The listing builds one solid part. Answer for the finished solid, in the listing's coordinates (mm). Face numbers are marked on the shaded views. A direction names the side the tool comes from. Give positions to 0.01 mm unless a question says otherwise; leave off trailing zeros. Order: outer loops, then holes, each group sorted by start corner. A loop starts at its lowest first (then second) coordinate and runs counter-clockwise, first axis right, second up. Notation, with made-up numbers: (51.5, 6.25) - (96.5, 6.25) arc R18 ccw to (96.5, 27.25) - close; hole circle Ø5 at (29, -26). An arc over 180 degrees is marked (long way). Answer as CSV lines item,"result". Start each with the question number.
1. Section D-D on x = 0.45 is taken. Give the vertices of the cut face in (y, z), and give its area (3 significant figures).
2. Section C-C on y = -2.5 is taken. Give the vertices of the cut face in (x, z), and give its area (3 significant figures).
3. Which of the six approach directions +Z, -Z, +X, -X, +Y, -Y give full straight-line access (tool end or side, diameter ignored) to the marked faces 1, 2, 3, 4 and 5?
4. Section B-B on x = 1.1 is taken. Give the vertices of the cut face in (y, z), and give its area (3 significant figures).
5. Consider line 1 along Z through (x, y) = (-0.7, -2.5); line 2 along Y through (x, z) = (-0.9, 2.95); line 3 along X through (y, z) = (3.5, 1.4). Determine where each line is inside the solid, lowest interval first. Write a range as [from, to].
6. Flat-ended cylindrical pins translate along their axes: pin 1 (0.8 mm diameter, centred on y = -3, z = 1.5, fed in from -X); pin 2 (1.2 mm diameter, centred on x = 0.5, y = 3, fed in from -Z); pin 3 (0.8 mm diameter, centred on y = 3, z = 1.5, fed in from +X). Find the tip coordinate at first contact, or state that the pin passes through.
7. Section A-A on z = 0.85 is taken. Give the vertices of the cut face in (x, y), and give its area (3 significant figures).
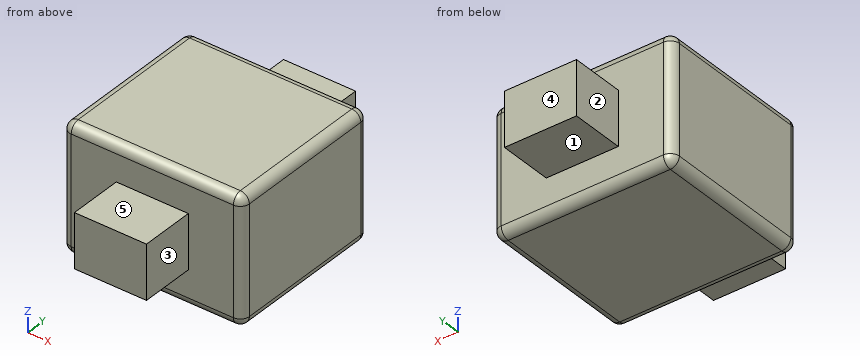
from build123d import *

# Parameters (mm, degrees)
SKETCH1_W           = 5
SKETCH1_H           = 4.5
BOSS_EXTRUDE1_DEPTH = 3.5
BOSS_EXTRUDE2_DEPTH = 1.5
BOSS_EXTRUDE3_DEPTH = 1.5
FILLET1_R           = 0.25


with BuildPart() as part:
    # Sketch1 → Boss-Extrude1 (new body)
    with BuildSketch(Plane.XY):
        Rectangle(SKETCH1_W, SKETCH1_H)
    extrude(amount=BOSS_EXTRUDE1_DEPTH)

    # Sketch2 → Boss-Extrude2 (add)
    with BuildSketch(Plane(origin=(0, 2.25, 0), x_dir=(1, 0, 0), z_dir=(0, 1, 0))):
        Polygon((-1, -2.45), (1, -1.05), (1, -1), (-1, -1), align=None)
        Polygon((1, -2.5), (1, -1.05), (-1, -2.45), (-1, -2.5), align=None)
    extrude(amount=BOSS_EXTRUDE2_DEPTH)

    # Sketch3 → Boss-Extrude3 (add)
    with BuildSketch(Plane(origin=(0, -2.25, 0), x_dir=(-1, 0, 0), z_dir=(0, -1, 0))):
        Polygon((-1, -1), (-1, -2.45), (1, -1.05), (1, -1), align=None)
        Polygon((1, -1.05), (-1, -2.45), (-1, -2.5), (1, -2.5), align=None)
    extrude(amount=BOSS_EXTRUDE3_DEPTH)

    # Fillet1
    fillet1_edges = [part.edges().sort_by_distance(p)[0] for p in [
        (-2.5, 0, 3.5),
        (0, -2.25, 3.5),
        (2.5, 0, 3.5),
        (0, -2.25, 0),
        (-2.5, 0, 0),
        (0, 2.25, 0),
        (2.5, 0, 0),
        (0, 2.25, 3.5),
        (2.5, -2.25, 1.75),
        (-2.5, -2.25, 1.75),
        (-2.5, 2.25, 1.75),
        (2.5, 2.25, 1.75),
    ]]
    fillet(fillet1_edges, radius=FILLET1_R)


solid = part.part
Checks:
1,outline,"(-3.75, 1) - (-2.25, 1) - (-2.25, 0.25) arc R0.25 ccw to (-2, 0) - (2, 0) arc R0.25 ccw to (2.25, 0.25) - (2.25, 1) - (3.75, 1) - (3.75, 2.5) - (2.25, 2.5) - (2.25, 3.25) arc R0.25 ccw to (2, 3.5) - (-2, 3.5) arc R0.25 ccw to (-2.25, 3.25) - (-2.25, 2.5) - (-3.75, 2.5) - close"
1,area,"20.2 mm²"
2,outline,"(-1, 1) - (1, 1) - (1, 2.5) - (-1, 2.5) - close"
2,area,"3.00 mm²"
3,face 1,"-Z, +X, -X, +Y"
3,face 2,"+Z, -Z, -X, +Y"
3,face 3,"+Z, -Z, +X, -Y"
3,face 4,"+Z, -Z, +X, -X, +Y"
3,face 5,"+Z, +X, -X, -Y"
4,outline,"(-2.25, 0.25) arc R0.25 ccw to (-2, 0) - (2, 0) arc R0.25 ccw to (2.25, 0.25) - (2.25, 3.25) arc R0.25 ccw to (2, 3.5) - (-2, 3.5) arc R0.25 ccw to (-2.25, 3.25) - close"
4,area,"15.7 mm²"
5,line 1,"z = [1, 2.5]"
5,line 2,"y = [-2.25, 2.25]"
5,line 3,"x = [-1, 1]"
6,pin 1,"stops at x = -1"
6,pin 2,"stops at z = 1"
6,pin 3,"stops at x = 1"
7,outline,"(-2.5, -2) arc R0.25 ccw to (-2.25, -2.25) - (2.25, -2.25) arc R0.25 ccw to (2.5, -2) - (2.5, 2) arc R0.25 ccw to (2.25, 2.25) - (-2.25, 2.25) arc R0.25 ccw to (-2.5, 2) - close"
7,area,"22.4 mm²"
